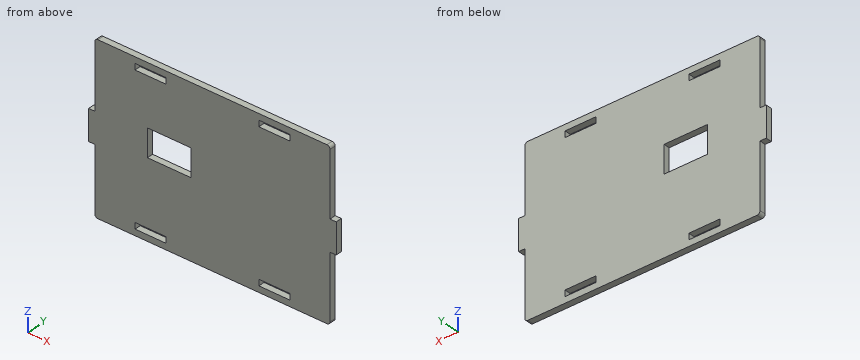
Solid Edge part; units mm, degrees
sketch "Sketch1" plane through (0, 0, 0) normal (0, -1, 0) x (1, 0, 0)
  line L0 (40, -27) -> (40, 27)
  line L1 (40, 27) -> (-40, 27)
  line L2 (-40, 27) -> (-40, -27)
  line L3 (-40, -27) -> (40, -27)
extrude "Protrusion1" add sketch "Sketch1" along normal blind 2
sketch "Sketch2" plane through (0, 0, 0) normal (0, -1, 0) x (1, 0, 0)
  line L0 (-25, 23) -> (-15, 23)
  line L1 (-15, 23) -> (-15, 25)
  line L2 (-15, 25) -> (-25, 25)
  line L3 (-25, 25) -> (-25, 23)
extrude "ExtrudedCutout_1" cut sketch "Sketch2" along normal blind 2
sketch "Sketch3" plane through (0, 0, 0) normal (0, -1, 0) x (1, 0, 0)
  line L0 (25, 25) -> (15, 25)
  line L1 (15, 25) -> (15, 23)
  line L2 (15, 23) -> (25, 23)
  line L3 (25, 23) -> (25, 25)
extrude "ExtrudedCutout_2" cut sketch "Sketch3" along normal blind 2
sketch "Sketch4" plane through (0, 0, 0) normal (0, -1, 0) x (1, 0, 0)
  line L0 (15, -25) -> (25, -25)
  line L1 (25, -25) -> (25, -23)
  line L2 (25, -23) -> (15, -23)
  line L3 (15, -23) -> (15, -25)
extrude "ExtrudedCutout_3" cut sketch "Sketch4" along normal blind 2
sketch "Sketch5" plane through (0, 0, 0) normal (0, -1, 0) x (1, 0, 0)
  line L0 (-15, -23) -> (-25, -23)
  line L1 (-25, -23) -> (-25, -25)
  line L2 (-25, -25) -> (-15, -25)
  line L3 (-15, -25) -> (-15, -23)
extrude "ExtrudedCutout_4" cut sketch "Sketch5" along normal blind 2
sketch "Sketch6" plane through (0, 0, 0) normal (0, -1, 0) x (1, 0, 0)
  line L0 (-38, -27) -> (-38, -5)
  line L1 (-38, -5) -> (-40, -5)
  line L2 (-40, -5) -> (-40, -27)
  line L3 (-40, -27) -> (-38, -27)
extrude "ExtrudedCutout_5" cut sketch "Sketch6" along normal blind 2
sketch "Sketch7" plane through (0, 0, 0) normal (0, -1, 0) x (1, 0, 0)
  line L0 (-38, 5) -> (-38, 27)
  line L1 (-38, 27) -> (-40, 27)
  line L2 (-40, 27) -> (-40, 5)
  line L3 (-40, 5) -> (-38, 5)
extrude "ExtrudedCutout_6" cut sketch "Sketch7" along normal blind 2
sketch "Sketch8" plane through (0, 0, 0) normal (0, -1, 0) x (1, 0, 0)
  line L0 (38, -5) -> (38, -27)
  line L1 (38, -27) -> (40, -27)
  line L2 (40, -27) -> (40, -5)
  line L3 (40, -5) -> (38, -5)
extrude "ExtrudedCutout_7" cut sketch "Sketch8" along normal blind 2
sketch "Sketch9" plane through (0, 0, 0) normal (0, -1, 0) x (1, 0, 0)
  line L0 (38, 27) -> (38, 5)
  line L1 (38, 5) -> (40, 5)
  line L2 (40, 5) -> (40, 27)
  line L3 (40, 27) -> (38, 27)
extrude "ExtrudedCutout_8" cut sketch "Sketch9" along normal blind 2
sketch "Sketch10" plane through (0, 0, 0) normal (0, -1, 0) x (1, 0, 0)
  line L0 (-21, -1.75) -> (-7, -1.75)
  line L1 (-7, -1.75) -> (-7, 7.25)
  line L2 (-7, 7.25) -> (-21, 7.25)
  line L3 (-21, 7.25) -> (-21, -1.75)
extrude "ExtrudedCutout_9" cut sketch "Sketch10" along normal blind 2
fillet "Round_1" radius 1 4 edges at (-38, -1, -27) (-38, -1, 27) (38, -1, 27) (38, -1, -27)
properties material "Acrylic, high impact grade"
Build history of the part. All positions in model axes, mm. Give positions to 0.01 mm unless a question says otherwise; leave off trailing zeros. Loops run counter-clockwise (first coordinate to the right, second up) from the corner with the lowest first, then second, coordinate; pieces in that order, holes last.
Item 1: Slice it at D-D, the plane z = 20.5. List the corners of the cut face in (x, y).
Answers follow:
outline: (-38, -2) - (38, -2) - (38, 0) - (-38, 0) - close
Item 2: Drill centre lines: line 1 (Z direction, x = 22, y = -1.5); line 2 (Z direction, x = -17.5, y = -1.45); line 3 (X direction, y = -1.4, z = -24). Where is each one in solid material? Low to high.
Answers follow:
line 1: z = -27 to -25, -23 to 23, 25 to 27
line 2: z = -27 to -25, -23 to -1.75, 7.25 to 23, 25 to 27
line 3: x = -38 to -25, -15 to 15, 25 to 38
Item 3: Slice it at B-B, the plane x = 17. List the corners of the cut face in (y, z).
Answers follow:
outline: (-2, -27) - (0, -27) - (0, -25) - (-2, -25) - close; (-2, -23) - (0, -23) - (0, 23) - (-2, 23) - close; (-2, 25) - (0, 25) - (0, 27) - (-2, 27) - close
Item 4: Slice it at C-C, the plane y = -0.65. Give the number of separate pieces and of enclosed holes in the cut face, and give its area (3 significant figures).
Answers follow:
separate pieces: 1
enclosed holes: 5
area: 3,940 mm2
Item 5: Slice it at A-A, the plane x = -19.5. List the corners of the cut face in (y, z), and give its area (3 significant figures).
Answers follow:
outline: (-2, -27) - (0, -27) - (0, -25) - (-2, -25) - close; (-2, -23) - (0, -23) - (0, -1.75) - (-2, -1.75) - close; (-2, 7.25) - (0, 7.25) - (0, 23) - (-2, 23) - close; (-2, 25) - (0, 25) - (0, 27) - (-2, 27) - close
area: 82.0 mm2
Item 6: Flat gauge pins, fed straight in: pin 1 (0.6 mm diameter, centred on x = -39, y = -1, fed in from -Z); pin 2 (0.6 mm diameter, centred on y = -1, z = -13, fed in from -X); pin 3 (0.6 mm diameter, centred on y = -1, z = -24.5, fed in from +X). Where does each tip first touch, or does it go through?
Answers follow:
pin 1: stops at z = -5
pin 2: stops at x = -38
pin 3: stops at x = 38
